```python
from build123d import *

# Parameters (mm, degrees)
BOSS_EXTRUDE1_DEPTH     = 2.54
SKETCH2_R               = 1.384838531
SKETCH2_R_2             = 1.27
CUT_EXTRUDE2_DEPTH      = 2.54
CUT_EXTRUDE4_DEPTH      = 7.62
CUT_EXTRUDE4_DEPTH_BACK = 10.16


with BuildPart() as part:
    # Sketch1 → Boss-Extrude1 (new body)
    with BuildSketch(Plane.XY):
        Polygon((-71.208440462, -3.308212961), (-24.728354348, 29.69264818), (-29.139739371, 35.905866523), (-75.619825485, 2.905005382), align=None)
    extrude(amount=BOSS_EXTRUDE1_DEPTH)

    # Sketch2 → Cut-Extrude2 (cut)
    with BuildSketch(Plane.XY.offset(2.54)):
        with Locations((-70.288529602, 2.017574604)):
            Circle(SKETCH2_R)
        with Locations((-30.065513702, 30.575915893)):
            Circle(SKETCH2_R_2)
    extrude(amount=-CUT_EXTRUDE2_DEPTH, mode=Mode.SUBTRACT)

    # Sketch3 → Cut-Extrude4 (cut, two sides)
    with BuildSketch(Plane(origin=(0, 0, 0), x_dir=(-1, 0, 0), z_dir=(0, 0, -1))) as cut_extrude4_sk:
        with BuildLine():
            Line((67.337713358, 2.689008108), (33.465419067, 26.769994698))
            ThreePointArc((33.465419067, 26.769994698), (33.166213405, 28.540948106), (34.937166813, 28.840153767))
            Line((34.937166813, 28.840153767), (68.809461104, 4.759167177))
            ThreePointArc((68.809461104, 4.759167177), (69.108666765, 2.988213769), (67.337713358, 2.689008108))
        make_face()
    extrude(amount=CUT_EXTRUDE4_DEPTH, mode=Mode.SUBTRACT)
    extrude(cut_extrude4_sk.sketch, amount=-CUT_EXTRUDE4_DEPTH_BACK, mode=Mode.SUBTRACT)


solid = part.part
```
Check sheet for the modelled part. Datum: model origin and axes. Units: mm. A direction names the side the tool comes from. Coordinates: 2 decimals unless noted, no trailing zeros. Order: outer loops, then holes, each group sorted by start corner. A loop starts at its lowest first (then second) coordinate and runs counter-clockwise, first axis right, second up. Notation, with made-up numbers: M 3,44 L 18,44 A8 cw 18,54 Z; hole C 71,20.25 d11. An arc over 180 degrees is marked long. One line per question, with ' | ' between items. Start each with the question number.
Item 1: Sectioned sample at C-C on z = 1.55. Record the cut outline in (x, y) (3 decimals), and give its area (3 significant figures).
Item 2: Access from +Z, -Z, +X, -X, +Y, -Y to the whole of each face (thin tool, end or side, straight path). Record for faces 1 (the flat face through (-50.64, 14.56, 1.25)), 2 (the flat face through (-48.294, 12.961, 1.252)).
Item 3: Material ranges on line 1 (X direction, y = 16.5, z = 1.55); line 2 (X direction, y = 11.5, z = 1.45); line 3 (Y direction, x = -55, z = 2.2), recorded low to high.
Item 4: Sectioned sample at B-B on x = -63. Record the cut outline in (y, z), and give its area (3 significant figures).
Item 5: Gauge pin test, flat ends, axial feed: P1, Ø1.5, axis at x = -43, z = 0.5, coming from the +Y side; P2, Ø1.5, axis at y = 27.5, z = 0.5, coming from the +X side; P3, Ø1.5, axis at x = -65, z = 2, coming from the -Y side; P4, Ø1.7, axis at x = -70.29, y = 2.02, coming from the +Z side. Record the tip position at first contact, or that the pin passes through.
Item 6: Mould release check, pull along X, two halves, no side actions. Record for faces 3 (the cylindrical face through (-28.854, 30.957, 1.288)), 4 (the cylindrical face through (-33.15, 28.52, 1.25)), 5 (the flat face through (-73.445, -0.158, 1.252)), 6 (the flat face through (-48, 15, 2.54)): pulls with the +X half, pulls with the -X half, needs draft (parallel to the pull), parting line crosses it, or undercut.
Item 7: Sectioned sample at A-A on y = 9. Record the cut outline in (x, z), and give its area (3 significant figures).
Answer below:
1) outline: M -75.62,2.905 L -71.208,-3.308 L -24.728,29.693 L -29.14,35.906 Z; hole C -70.289,2.018 d2.77; hole M -68.809,4.759 A1.27 ccw -67.338,2.689 L -33.465,26.77 A1.27 ccw -34.937,28.84 Z; hole C -30.066,30.576 d2.54 | area: 313 mm^2
2) face 1: +Z, -Z | face 2: +Z, -Z, +X, -Y
3) line 1: x = -56.47 to -52.29, -47.91 to -43.31 | line 2: x = -63.51 to -59.33, -54.94 to -50.35 | line 3: y = 8.2 to 11.46, 14.58 to 17.55
4) outline: M 2.52,0 L 5.77,0 L 5.77,2.54 L 2.52,2.54 Z; M 8.89,0 L 11.87,0 L 11.87,2.54 L 8.89,2.54 Z | area: 15.8 mm^2
5) P1: stops at y = 26.6 | P2: stops at x = -26.76 | P3: stops at y = 0.57 | P4: passes through
6) face 3: undercut | face 4: undercut | face 5: pulls with the -X half | face 6: needs draft
7) outline: M -67.04,0 L -62.84,0 L -62.84,2.54 L -67.04,2.54 Z; M -58.46,0 L -53.87,0 L -53.87,2.54 L -58.46,2.54 Z | area: 22.3 mm^2
